Geometry: final body of the model. Coordinates: model frame, mm. Round coordinates to 2 decimals unless told otherwise and drop trailing zeros. Order: outer loops, then holes, each group sorted by start corner. A loop starts at its lowest first (then second) coordinate and runs counter-clockwise, first axis right, second up. Notation, with made-up numbers: (84, -34) -> (116, -34) arc R27 ccw to (116, -6) -> close; hole circle Ø1 at (-5.75, -2.5). An arc over 180 degrees is marked (long way). Put each result on its own line as item: value.
Autodesk Inventor part; units mm, degrees
ref_plane "YZ Plane" through (0, 0, 0) normal (1, 0, 0) x (0, 1, 0)
ref_plane "XZ Plane" through (0, 0, 0) normal (0, 1, 0) x (-1, 0, 0)
ref_plane "XY Plane" through (0, 0, 0) normal (0, 0, 1) x (1, 0, 0)
sketch "Sketch1" plane through (0, 0, 0) normal (0, 0, 1) x (1, 0, 0)
  line L0 (77.1826, 34.3167) -> (88.1826, 34.3167)
  line L1 (88.6826, 33.8167) -> (88.6826, 17.8167)
  line L2 (88.1826, 17.3167) -> (77.1826, 17.3167)
  line L3 (76.6826, 17.8167) -> (76.6826, 33.8167)
  arc A0 (77.1826, 34.3167) -> (76.6826, 33.8167) centre (77.1826, 33.8167) ccw
  arc A1 (88.6826, 33.8167) -> (88.1826, 34.3167) centre (88.1826, 33.8167) ccw
  arc A2 (88.1826, 17.3167) -> (88.6826, 17.8167) centre (88.1826, 17.8167) ccw
  arc A3 (76.6826, 17.8167) -> (77.1826, 17.3167) centre (77.1826, 17.8167) ccw
  line L4 (82.4065, 34.3167) -> (82.6826, 17.3167)
  point P0 (0, 0)
  point P1 (88.6826, 17.3167)
  point P2 (88.6826, 34.3167)
  point P3 (76.6826, 17.3167)
  dimension "d0" = 12
  dimension "d1" = 17
  dimension "d2" = 0.5
extrude "Extrusion1" add sketch "Sketch1" along normal blind 2
sketch "Sketch2" plane through (0, 0, 2) normal (0, 0, 1) x (1, 0, 0)
  point P0 (0, 0)
  point P1 (82.7526, 32.5302)
hole "Hole1" at (82.7526, 32.5302, 2) direction (0, 0, -1) diameter 3 depth 55.5
sketch "Sketch3" plane through (0, 0, 2) normal (0, 0, 1) x (1, 0, 0)
  point P0 (0, 0)
  point P1 (82.7236, 19.0448)
hole "Hole2" at (82.7236, 19.0448, 2) direction (0, 0, -1) diameter 3 depth 55.5
sketch "Sketch5" plane through (0, 0, 0) normal (0, 0, 1) x (1, 0, 0)
  line L0 (88.1826, 34.3167) -> (77.1826, 34.3167)
  line L1 (77.1826, 17.3167) -> (88.1826, 17.3167)
  line L2 (83.824, 30.7891) -> (81.5769, 30.7891) construction
  line L3 (81.5769, 30.7891) -> (81.5769, 20.7942) construction
  line L4 (81.5769, 20.7942) -> (83.824, 20.7942) construction
  line L5 (83.824, 20.7942) -> (83.824, 30.7891) construction
  point P0 (0, 0)
properties part number "termo" material "Wood (Oak)"
1. Contact query for a flat-ended pin moving along its axis: P1, Ø2.5, axis at x = 82.75, y = 32.53, coming from the -Z side. Output: stop coordinate, or through.
Ans:
P1: through
2. Draft query along Y for faces 1 (the face through (83, 17.317, 1)), 2 (the face through (84.083, 31.838, 0.986)), 3 (the face through (88.683, 26, 1)). Return one class per face: +Y half, -Y half, draft (parallel to the pull), parting line (faces both ways), or undercut.
Ans:
face 1: -Y half
face 2: undercut
face 3: draft
3. Cut plane C-C on z = 0.65. Return loops of the section in (x, y), and give its area (3 significant figures).
Ans:
outline: (76.68, 17.82) arc R0.5 ccw to (77.18, 17.32) -> (88.18, 17.32) arc R0.5 ccw to (88.68, 17.82) -> (88.68, 33.82) arc R0.5 ccw to (88.18, 34.32) -> (77.18, 34.32) arc R0.5 ccw to (76.68, 33.82) -> close; hole circle Ø3 at (82.72, 19.04); hole circle Ø3 at (82.75, 32.53)
area: 190 mm²
4. Cut plane B-B on x = 84. Return loops of the section in (y, z), and give its area (3 significant figures).
Ans:
outline: (17.32, 0) -> (18.26, 0) -> (18.26, 2) -> (17.32, 2) -> close; (19.83, 0) -> (31.7, 0) -> (31.7, 2) -> (19.83, 2) -> close; (33.36, 0) -> (34.32, 0) -> (34.32, 2) -> (33.36, 2) -> close
area: 27.5 mm²
5. Cut plane D-D on x = 82. Return loops of the section in (y, z).
Ans:
outline: (17.32, 0) -> (17.73, 0) -> (17.73, 2) -> (17.32, 2) -> close; (20.36, 0) -> (31.23, 0) -> (31.23, 2) -> (20.36, 2) -> close; (33.83, 0) -> (34.32, 0) -> (34.32, 2) -> (33.83, 2) -> close
6. Material intervals for probe 1 along Y at (x, z) = (84, 0.9); probe 2 along Y at (x, z) = (82.25, 0.3); probe 3 along X at (y, z) = (19.5, 0.7), sorted ascending.
Ans:
probe 1: 17.32 to 18.26, 19.83 to 31.7, 33.36 to 34.32
probe 2: 17.32 to 17.62, 20.47 to 31.12, 33.94 to 34.32
probe 3: 76.68 to 81.29, 84.15 to 88.68
7. Cut plane A-A on y = 19.75. Return loops of the section in (x, z), and give its area (3 significant figures).
Ans:
outline: (76.68, 0) -> (81.4, 0) -> (81.4, 2) -> (76.68, 2) -> close; (84.05, 0) -> (88.68, 0) -> (88.68, 2) -> (84.05, 2) -> close
area: 18.7 mm²
